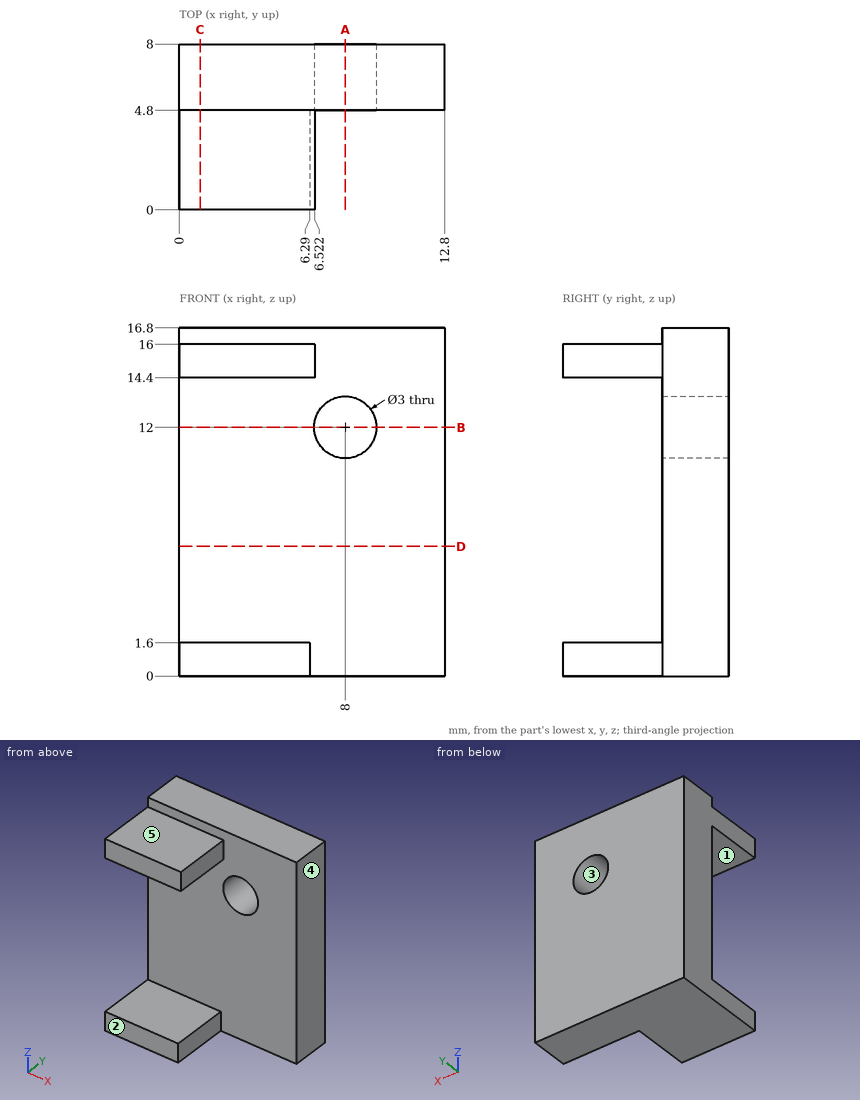
Source: three-view drawing plus pictorial views. Frame: mm from the lowest corner of the part. A direction names the side the tool comes from. Coordinates: 2 decimals unless noted, no trailing zeros. Loops run counter-clockwise (first coordinate to the right, second up) from the corner with the lowest first, then second, coordinate; pieces in that order, holes last. Notation, with made-up numbers: (27, -21.5) -> (43, -21.5) arc R17 ccw to (43, 8.5) -> close; hole circle Ø1 at (70.5, 58.25). An arc over 180 degrees is marked (long way). Answer in a Markdown table with one row per item. Add a question column.
Q1. Section D-D on z = 6.25. Return the cut outline in (x, y).
Q2. Section B-B on z = 12. Return the cut outline in (x, y).
Q3. Contact query for flat-ended pins moving along their axis: pin 1 Ø0.8 at (y, z) = (2.5, 15) entering from +X; pin 2 Ø4 at (x, y) = (1.5, 2) entering from +Z; pin 3 Ø3 at (x, z) = (5, 5) entering from -Y. Output: stop coordinate, or through.
Q4. Pull-direction query (Z, two-part tool) for the marked faces 3, 4 and 5; classes: pulls with the +Z half, pulls with the -Z half, needs draft (parallel to the pull), parting line crosses it, or undercut.
Q5. Section A-A on x = 8. Return the cut outline in (y, z).
Q6. Section C-C on x = 1. Return the cut outline in (y, z).
Q7. Reachability of the marked faces 1 and 2 from +Z, -Z, +X, -X, +Y, -Y: full face, straight path, thin tool, end or side. Return the list, or none.
Q8. Ray query, line 1 along Z through (x, y) = (3.75, 4); line 2 along X through (y, z) = (6.35, 12); line 3 along Y through (x, z) = (2.75, 9). Return the intervals inside material, ascending.
Computed values:
| question | item | result |
|---|---|---|
| 1 | outline | (0, 4.8) -> (12.8, 4.8) -> (12.8, 8) -> (0, 8) -> close |
| 2 | outline | (0, 4.8) -> (6.5, 4.8) -> (6.5, 8) -> (0, 8) -> close; (9.5, 4.8) -> (12.8, 4.8) -> (12.8, 8) -> (9.5, 8) -> close |
| 3 | pin 1 | stops at x = 6.52 |
| 3 | pin 2 | stops at z = 16 |
| 3 | pin 3 | stops at y = 4.8 |
| 4 | face 3 | undercut |
| 4 | face 4 | needs draft |
| 4 | face 5 | pulls with the +Z half |
| 5 | outline | (4.8, 0) -> (8, 0) -> (8, 10.5) -> (4.8, 10.5) -> close; (4.8, 13.5) -> (8, 13.5) -> (8, 16.8) -> (4.8, 16.8) -> close |
| 6 | outline | (0, 0) -> (8, 0) -> (8, 16.8) -> (4.8, 16.8) -> (4.8, 16) -> (0, 16) -> (0, 14.4) -> (4.8, 14.4) -> (4.8, 1.6) -> (0, 1.6) -> close |
| 7 | face 1 | +X, -X, -Y |
| 7 | face 2 | +Z, -Z, +X, -X, -Y |
| 8 | line 1 | z = 0 to 1.6, 14.4 to 16 |
| 8 | line 2 | x = 0 to 6.5, 9.5 to 12.8 |
| 8 | line 3 | y = 4.8 to 8 |
